```python
from build123d import *

# Parameters (mm, degrees)
BOSS_EXTRUDE1_DEPTH = 1.5
SKETCH2_R           = 10.5
BOSS_EXTRUDE2_DEPTH = 10
SKETCH3_R           = 9
CUT_EXTRUDE1_DEPTH  = 24


with BuildPart() as part:
    # Sketch1 → Boss-Extrude1 (new body, symmetric)
    with BuildSketch(Plane(origin=(0, 0, 0), x_dir=(1, 0, 0), z_dir=(0, 1, 0))):
        Polygon((6.350852961, -11), (12.701705922, 0), (6.350852961, 11), (-6.350852961, 11), (-12.701705922, 0), (-6.350852961, -11), align=None)
    extrude(amount=BOSS_EXTRUDE1_DEPTH, both=True)

    # Sketch2 → Boss-Extrude2 (add)
    with BuildSketch(Plane(origin=(0, 1.5, 0), x_dir=(1, 0, 0), z_dir=(0, 1, 0))):
        Circle(SKETCH2_R)
    boss_extrude2 = extrude(amount=BOSS_EXTRUDE2_DEPTH)

    # Mirror1: Boss-Extrude2 across plane
    add(boss_extrude2.mirror(Plane.ZX))

    # Sketch3 → Cut-Extrude1 (cut, through all)
    with BuildSketch(Plane(origin=(0, 11.5, 0), x_dir=(1, 0, 0), z_dir=(0, 1, 0))):
        Circle(SKETCH3_R)
    extrude(amount=-CUT_EXTRUDE1_DEPTH, mode=Mode.SUBTRACT)


solid = part.part
```
Part model, mm, in its own coordinate system. A direction names the side the tool comes from. Round coordinates to 2 decimals unless told otherwise and drop trailing zeros. Write each loop counter-clockwise with the first axis right and the second up, starting at its lowest first coordinate (ties: lowest second). Pieces come first, ordered by that corner, then holes.
Item 1: Cut at B-B, the plane z = 7.25. Give the cut face in (x, y).
Results:
outline: (-8.52, -1.5) - (-7.6, -1.5) - (-7.6, -11.5) - (-5.33, -11.5) - (-5.33, 11.5) - (-7.6, 11.5) - (-7.6, 1.5) - (-8.52, 1.5) - close; (5.33, -11.5) - (7.6, -11.5) - (7.6, -1.5) - (8.52, -1.5) - (8.52, 1.5) - (7.6, 1.5) - (7.6, 11.5) - (5.33, 11.5) - close
Item 2: Cut at A-A, the plane x = 0. Give the cut face in (y, z).
Results:
outline: (-11.5, -10.5) - (-1.5, -10.5) - (-1.5, -11) - (1.5, -11) - (1.5, -10.5) - (11.5, -10.5) - (11.5, -9) - (-11.5, -9) - close; (-11.5, 9) - (11.5, 9) - (11.5, 10.5) - (1.5, 10.5) - (1.5, 11) - (-1.5, 11) - (-1.5, 10.5) - (-11.5, 10.5) - close
Item 3: Probe L1, parallel to Z at x = 0, y = 5.25; L2, parallel to Z at x = -5.5, y = 10. List the from-to ranges inside material, lowest first.
Results:
L1: z = -10.5 to -9, 9 to 10.5
L2: z = -8.94 to -7.12, 7.12 to 8.94
Item 4: Drop flat-ended pins along their axis: pin 1 Ø2 at (x, y) = (-7, -9) entering from +Z; pin 2 Ø6 at (x, z) = (0, -4.5) entering from -Y; pin 3 Ø1 at (y, z) = (-2.5, 2) entering from -X; pin 4 Ø3 at (y, z) = (-7, 7.5) entering from +X. Give the stop position or say it passes through.
Results:
pin 1: stops at z = 8.62
pin 2: passes through
pin 3: stops at x = -10.39
pin 4: stops at x = 8.62
Item 5: Cut at C-C, the plane y = -7.5. Give the cut face in (x, z), plus the area to 3 significant figures.
Results:
outline: circle Ø21 at (0, 0); hole circle Ø18 at (0, 0)
area: 91.9 mm2
Item 6: Which spindle directions (+Z, -Z, +X, -X, +Y, -Y) get a long thin tool onto all of the face, cutting with end or side? Do faces 1 (the flat face through (8, 11.5, -5)), 2 (the flat face through (10.3, -1.5, 3.2)), 3 (the flat face through (10.3, 1.5, 3.2)). Say none if no direction does.
Results:
face 1: +Z, -Z, +X, -X, +Y
face 2: -Y
face 3: +Y
Item 7: Two-plate mould, pull along Z, no slides. Class faces 4 (the cylindrical face through (-1.172, 0.161, -8.923)), 5 (the flat face through (0, 0, -11)), 6 (the cylindrical face through (10, -6.4, -3.2)): +Z half, -Z half, draft (parallel to the pull), parting line (faces both ways), or undercut.
Results:
face 4: undercut
face 5: -Z half
face 6: parting line
